Geometry check sheet. Reference: the model listing, model coordinates, mm. A direction names the side the tool comes from. Round coordinates to 2 decimals unless told otherwise and drop trailing zeros. Order: outer loops, then holes, each group sorted by start corner. A loop starts at its lowest first (then second) coordinate and runs counter-clockwise, first axis right, second up.
(1) Sectioned sample at C-C (z = -1). Record the boundary of the cut face in (x, y), plus the area to 3 significant figures.
(2) Go/stop test with flat-tipped pins: pin 1 (4 mm diameter, centred on y = -3.5, z = -5.5, fed in from -X); pin 2 (2.5 mm diameter, centred on x = 1.5, y = -4.5, fed in from +Z); pin 3 (2.5 mm diameter, centred on x = -5, y = -3.5, fed in from -Z). Record where each tip stops, or that it passes through.
(3) Release check for a two-part mould opening along Z. For faces 4 (the face through (-6.698, 0.089, -6.176)), 5 (the face through (0, 0, -14.954)), 6 (the face through (-13.367, -4, 0)) record: +Z half, -Z half, draft (parallel to the pull), parting line (faces both ways), or undercut.
(4) Material ranges on line 1 along X through (y, z) = (-3, 9.5); line 2 along Z through (x, y) = (7, -3.5); line 3 along X through (y, z) = (-5, -10.75), recorded low to high.
(5) Sectioned sample at A-A (y = 4.5). Record the boundary of the cut face in (x, z), plus the area to 3 significant figures.
(6) Set-up check for faces 1 (the face through (-6, 6.35, -6)), 2 (the face through (4.2, 0.1, -7.1)), 3 (the face through (13.367, -4, 0)): record each of +Z, -Z, +X, -X, +Y, -Y from which the full face is reachable in a straight line by a thin tool's end or side.
(7) Sectioned sample at D-D (x = -2.5). Record the boundary of the cut face in (y, z).
(8) Sectioned sample at B-B (x = 8.75). Record the boundary of the cut face in (y, z).
from build123d import *

# Parameters (mm, degrees)
SKETCH1_W           = 26.7335
SKETCH1_H           = 26.7335
BOSS_EXTRUDE1_DEPTH = 6.35
SKETCH2_W           = 29.9085
SKETCH2_H           = 29.9085
BOSS_EXTRUDE2_DEPTH = 1.4605
CUT_EXTRUDE1_DEPTH  = 13.7


with BuildPart() as part:
    # Sketch1 → Boss-Extrude1 (new body, symmetric)
    with BuildSketch(Plane(origin=(0, 0, 0), x_dir=(1, 0, 0), z_dir=(0, 1, 0))):
        Rectangle(SKETCH1_W, SKETCH1_H)
    extrude(amount=BOSS_EXTRUDE1_DEPTH, both=True)

    # Sketch2 → Boss-Extrude2 (add, symmetric)
    with BuildSketch(Plane(origin=(0, 0, 0), x_dir=(1, 0, 0), z_dir=(0, 1, 0))):
        Rectangle(SKETCH2_W, SKETCH2_H)
    extrude(amount=BOSS_EXTRUDE2_DEPTH, both=True)

    # Sketch3 → Cut-Extrude1 (cut, through all)
    with BuildSketch(Plane(origin=(0, 6.35, 0), x_dir=(1, 0, 0), z_dir=(0, 1, 0))):
        with BuildLine():
            Line((-2, 9.797958971), (-2, 8.003905297))
            ThreePointArc((-2, 8.003905297), (-4.125, 7.144709581), (-5.931585317, 5.734003456))
            Line((-5.931585317, 5.734003456), (-7.485281374, 6.631030293))
            ThreePointArc((-7.485281374, 6.631030293), (-8.660254038, 5), (-9.485281374, 3.166928678))
            Line((-9.485281374, 3.166928678), (-7.931585317, 2.269901841))
            ThreePointArc((-7.931585317, 2.269901841), (-8.25, 0), (-7.931585317, -2.269901841))
            Line((-7.931585317, -2.269901841), (-9.485281374, -3.166928678))
            ThreePointArc((-9.485281374, -3.166928678), (-8.660254038, -5), (-7.485281374, -6.631030293))
            Line((-7.485281374, -6.631030293), (-5.931585317, -5.734003456))
            ThreePointArc((-5.931585317, -5.734003456), (-4.125, -7.144709581), (-2, -8.003905297))
            Line((-2, -8.003905297), (-2, -9.797958971))
            ThreePointArc((-2, -9.797958971), (0, -10), (2, -9.797958971))
            Line((2, -9.797958971), (2, -8.003905297))
            ThreePointArc((2, -8.003905297), (4.125, -7.144709581), (5.931585317, -5.734003456))
            Line((5.931585317, -5.734003456), (7.485281374, -6.631030293))
            ThreePointArc((7.485281374, -6.631030293), (8.660254038, -5), (9.485281374, -3.166928678))
            Line((9.485281374, -3.166928678), (7.931585317, -2.269901841))
            ThreePointArc((7.931585317, -2.269901841), (8.25, 0), (7.931585317, 2.269901841))
            Line((7.931585317, 2.269901841), (9.485281374, 3.166928678))
            ThreePointArc((9.485281374, 3.166928678), (8.660254038, 5), (7.485281374, 6.631030293))
            Line((7.485281374, 6.631030293), (5.931585317, 5.734003456))
            ThreePointArc((5.931585317, 5.734003456), (4.125, 7.144709581), (2, 8.003905297))
            Line((2, 8.003905297), (2, 9.797958971))
            ThreePointArc((2, 9.797958971), (0, 10), (-2, 9.797958971))
        make_face()
    extrude(amount=-CUT_EXTRUDE1_DEPTH, mode=Mode.SUBTRACT)


solid = part.part
Answer below:
1. outline: (-14.95, -1.46) - (-13.37, -1.46) - (-13.37, -6.35) - (-8.19, -6.35) - (-8.19, 6.35) - (-13.37, 6.35) - (-13.37, 1.46) - (-14.95, 1.46) - close; (8.19, -6.35) - (13.37, -6.35) - (13.37, -1.46) - (14.95, -1.46) - (14.95, 1.46) - (13.37, 1.46) - (13.37, 6.35) - (8.19, 6.35) - close
1. area: 141 mm2
2. pin 1: stops at x = -13.37
2. pin 2: stops at z = 13.37
2. pin 3: stops at z = -13.37
3. face 4: undercut
3. face 5: -Z half
3. face 6: draft
4. line 1: x = -13.37 to -2, 2 to 13.37
4. line 2: z = -13.37 to -6.35, 6.35 to 13.37
4. line 3: x = -13.37 to 13.37
5. outline: (-13.37, -13.37) - (13.37, -13.37) - (13.37, 13.37) - (-13.37, 13.37) - close; hole (-9.49, -3.17) arc R10 ccw to (-7.49, -6.63) - (-5.93, -5.73) arc R8.25 ccw to (-2, -8) - (-2, -9.8) arc R10 ccw to (2, -9.8) - (2, -8) arc R8.25 ccw to (5.93, -5.73) - (7.49, -6.63) arc R10 ccw to (9.49, -3.17) - (7.93, -2.27) arc R8.25 ccw to (7.93, 2.27) - (9.49, 3.17) arc R10 ccw to (7.49, 6.63) - (5.93, 5.73) arc R8.25 ccw to (2, 8) - (2, 9.8) arc R10 ccw to (-2, 9.8) - (-2, 8) arc R8.25 ccw to (-5.93, 5.73) - (-7.49, 6.63) arc R10 ccw to (-9.49, 3.17) - (-7.93, 2.27) arc R8.25 ccw to (-7.93, -2.27) - close
5. area: 459 mm2
6. face 1: +Z, -Z, +X, -X, +Y
6. face 2: +Y, -Y
6. face 3: +Z, -Z, +X, -Y
7. outline: (-6.35, -13.37) - (-1.46, -13.37) - (-1.46, -14.95) - (1.46, -14.95) - (1.46, -13.37) - (6.35, -13.37) - (6.35, -7.86) - (-6.35, -7.86) - close; (-6.35, 7.86) - (6.35, 7.86) - (6.35, 13.37) - (1.46, 13.37) - (1.46, 14.95) - (-1.46, 14.95) - (-1.46, 13.37) - (-6.35, 13.37) - close
8. outline: (-6.35, -13.37) - (-1.46, -13.37) - (-1.46, -14.95) - (1.46, -14.95) - (1.46, -13.37) - (6.35, -13.37) - (6.35, -4.84) - (-6.35, -4.84) - close; (-6.35, -2.74) - (6.35, -2.74) - (6.35, 2.74) - (-6.35, 2.74) - close; (-6.35, 4.84) - (6.35, 4.84) - (6.35, 13.37) - (1.46, 13.37) - (1.46, 14.95) - (-1.46, 14.95) - (-1.46, 13.37) - (-6.35, 13.37) - close
